from build123d import *

# Parameters (mm, degrees)
F0_W      = 33.02
F0_H      = 33.02
F1_DEPTH  = 127
F2_W      = 30.48
F2_H      = 30.48
F3_DEPTH  = 127
F4_W      = 25.4
F4_H      = 33.02
F4_R      = 6.35
F5_DEPTH  = 33.02
F6_W      = 30.48
F6_H      = 33.02
F7_DEPTH  = 25.4
F8_W      = 12.7
F8_H      = 12.7
F8_R      = 3.175
F9_DEPTH  = 33.02
F10_W     = 26.4536738396
F10_H     = 12.7
F11_DEPTH = 12.7


with BuildPart() as f1:
    # F0 (on Front) → F1 (new body)
    with BuildSketch(Plane.XZ):
        Rectangle(F0_W, F0_H)
    extrude(amount=F1_DEPTH)

    # F2 (on face) → F3 (cut)
    with BuildSketch(Plane.XZ.offset(127)):
        Rectangle(F2_W, F2_H)
    extrude(amount=-F3_DEPTH, mode=Mode.SUBTRACT)

    # F4 (on face) → F5 (join)
    with BuildSketch(Plane.YZ.offset(16.51)):
        with Locations((12.7, 0)):
            Rectangle(F4_W, F4_H)
        with Locations((12.7, 0)):
            Circle(F4_R, mode=Mode.SUBTRACT)
    extrude(amount=-F5_DEPTH)

    # F6 (on face) → F7 (cut)
    with BuildSketch(Plane(origin=(0, 25.4, 0), x_dir=(-1, 0, 0), z_dir=(0, 1, 0))):
        Rectangle(F6_W, F6_H)
    extrude(amount=-F7_DEPTH, mode=Mode.SUBTRACT)

    # F8 (on face) → F9 (join)
    with BuildSketch(Plane.YZ.offset(16.51)):
        with Locations((-19.05, -22.86)):
            Rectangle(F8_W, F8_H)
        with Locations((-19.05, -22.86)):
            Circle(F8_R, mode=Mode.SUBTRACT)
    extrude(amount=-F9_DEPTH)

    # F10 (on face) → F11 (cut)
    with BuildSketch(Plane(origin=(0, 0, -29.21), x_dir=(1, 0, 0), z_dir=(0, 0, -1))):
        with Locations((-0.37084613, 19.05)):
            Rectangle(F10_W, F10_H)
    extrude(amount=-F11_DEPTH, mode=Mode.SUBTRACT)


solid = f1.part
Geometry: final body of the model. Coordinates: model frame, mm. A direction names the side the tool comes from. Coordinates: 2 decimals unless noted, no trailing zeros. Order: outer loops, then holes, each group sorted by start corner. A loop starts at its lowest first (then second) coordinate and runs counter-clockwise, first axis right, second up.
1) First-contact query: P1, Ø1, axis at x = -7.5, z = -16, coming from the +Y side; P2, Ø1.8, axis at x = 14.5, z = -25, coming from the +Y side; P3, Ø2.5, axis at x = -14.5, z = -22, coming from the -Y side; P4, Ø16.5, axis at x = 8, y = -17, coming from the -Z side. Flat tips, straight axial feed; report the tip coordinate or a pass-through.
Result sheet:
P1: stops at y = 0
P2: stops at y = -12.7
P3: stops at y = -25.4
P4: stops at z = -29.21
2) Ray query, probe 1 along Z at (x, y) = (-14, -19); probe 2 along X at (y, z) = (-89, -4.5). Return the intervals inside material, ascending.
Result sheet:
probe 1: z = -29.21 to -26.03, -19.69 to -15.24, 15.24 to 16.51
probe 2: x = -16.51 to -15.24, 15.24 to 16.51
3) Section B-B (z = 0). Return loops of the section in (x, y).
Result sheet:
outline: (-16.51, -127) - (-15.24, -127) - (-15.24, 6.35) - (-16.51, 6.35) - close; (-16.51, 19.05) - (-15.24, 19.05) - (-15.24, 25.4) - (-16.51, 25.4) - close; (15.24, -127) - (16.51, -127) - (16.51, 6.35) - (15.24, 6.35) - close; (15.24, 19.05) - (16.51, 19.05) - (16.51, 25.4) - (15.24, 25.4) - close
4) Section D-D (y = 12.7). Return loops of the section in (x, z).
Result sheet:
outline: (-16.51, -16.51) - (-15.24, -16.51) - (-15.24, -6.35) - (-16.51, -6.35) - close; (-16.51, 6.35) - (-15.24, 6.35) - (-15.24, 16.51) - (-16.51, 16.51) - close; (15.24, -16.51) - (16.51, -16.51) - (16.51, -6.35) - (15.24, -6.35) - close; (15.24, 6.35) - (16.51, 6.35) - (16.51, 16.51) - (15.24, 16.51) - close
5) Section A-A (y = -19.05). Return loops of the section in (x, z) (3 decimals), then the cut area to 3 significant figures.
Result sheet:
outline: (-16.51, -29.21) - (-13.598, -29.21) - (-13.598, -26.035) - (-16.51, -26.035) - close; (-16.51, -19.685) - (-13.598, -19.685) - (-13.598, -16.51) - (12.856, -16.51) - (12.856, -19.685) - (16.51, -19.685) - (16.51, 16.51) - (-16.51, 16.51) - close; (12.856, -29.21) - (16.51, -29.21) - (16.51, -26.035) - (12.856, -26.035) - close; hole (-15.24, -15.24) - (15.24, -15.24) - (15.24, 15.24) - (-15.24, 15.24) - close
area: 203 mm2
6) Set-up query: faces 4 (the flat face through (-15, -12.7, -23)), 5 (the flat face through (0, -64, 15.24)), 6 (the flat face through (-15, -25.4, -23)). Return all of +Z, -Z, +X, -X, +Y, -Y with unobstructed straight access to the full face (end or side cutting, diameter ignored); none if empty.
Result sheet:
face 4: -Z, +X, -X, +Y
face 5: +Y, -Y
face 6: -Z, +X, -X, -Y
7) Section C-C (x = 3). Return loops of the section in (y, z), then the cut area to 3 significant figures.
Result sheet:
outline: (-127, -16.51) - (0, -16.51) - (0, -15.24) - (-127, -15.24) - close; (-127, 15.24) - (0, 15.24) - (0, 16.51) - (-127, 16.51) - close
area: 323 mm2
8) Draft query along Z for faces 1 (the cylindrical face through (15.884, 6.356, 0.279)), 2 (the flat face through (15, -19, -29.21)), 3 (the flat face through (-13.598, -16.1, -24.4)). Return one class per face: released by +Z, released by -Z, zero draft, split by the parting line, or undercut.
Result sheet:
face 1: undercut
face 2: released by -Z
face 3: zero draft
